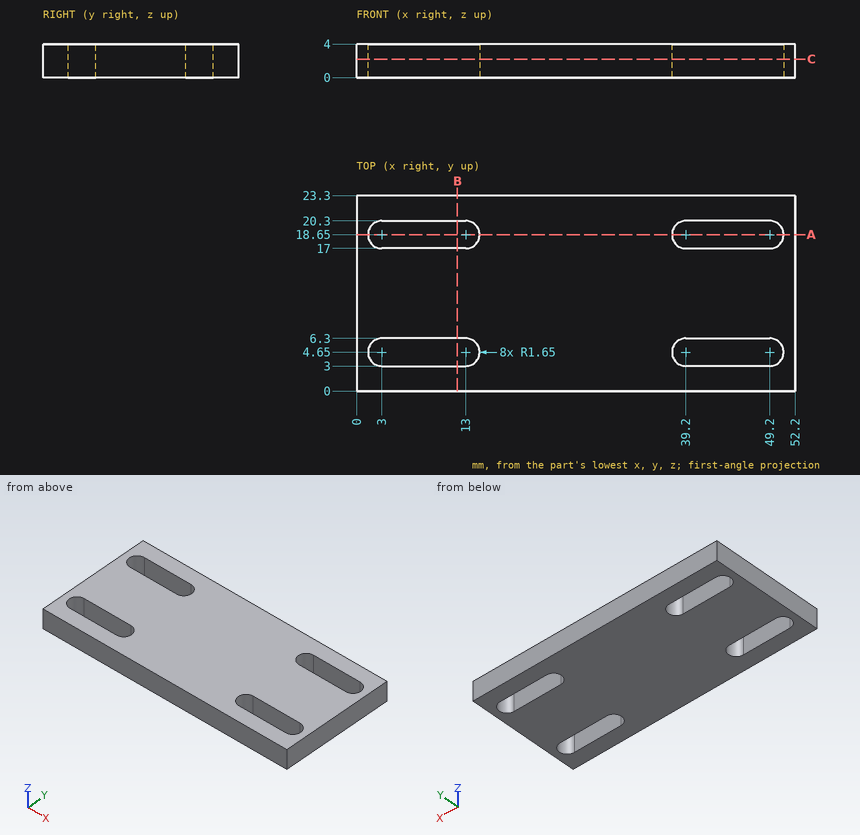
Print and shaded views of the part. All mm, measured from the part's lowest x, y and z. Give positions to 0.01 mm unless a question says otherwise; leave off trailing zeros. Loops run counter-clockwise (first coordinate to the right, second up) from the corner with the lowest first, then second, coordinate; pieces in that order, holes last.
1) Wall check: line 1 (Y direction, x = 6, z = 3.2); line 2 (Y direction, x = 38, z = 0.7). Give the ranges that are in metal, low to high.
2) Saw through at B-B (x = 12). Write the cut outline in (y, z).
3) Saw through at A-A (y = 18.65). Write the cut outline in (x, z), plus the area to 3 significant figures.
4) Saw through at C-C (z = 2.2). Write the cut outline in (x, y).
Answer block:
1. line 1: y = 0 to 3, 6.3 to 17, 20.3 to 23.3
1. line 2: y = 0 to 3.52, 5.78 to 17.52, 19.78 to 23.3
2. outline: (0, 0) - (3, 0) - (3, 4) - (0, 4) - close; (6.3, 0) - (17, 0) - (17, 4) - (6.3, 4) - close; (20.3, 0) - (23.3, 0) - (23.3, 4) - (20.3, 4) - close
3. outline: (0, 0) - (1.35, 0) - (1.35, 4) - (0, 4) - close; (14.65, 0) - (37.55, 0) - (37.55, 4) - (14.65, 4) - close; (50.85, 0) - (52.2, 0) - (52.2, 4) - (50.85, 4) - close
3. area: 102 mm2
4. outline: (0, 0) - (52.2, 0) - (52.2, 23.3) - (0, 23.3) - close; hole (3, 3) - (13, 3) arc R1.65 ccw to (13, 6.3) - (3, 6.3) arc R1.65 ccw to start; hole (3, 17) - (13, 17) arc R1.65 ccw to (13, 20.3) - (3, 20.3) arc R1.65 ccw to start; hole (39.2, 3) - (49.2, 3) arc R1.65 ccw to (49.2, 6.3) - (39.2, 6.3) arc R1.65 ccw to start; hole (39.2, 17) - (49.2, 17) arc R1.65 ccw to (49.2, 20.3) - (39.2, 20.3) arc R1.65 ccw to start
